Study the drawing (mm; zero at the part's minimum x, y, z) and answer. A direction names the side the tool comes from. Coordinates: 2 decimals unless noted, no trailing zeros. Order: outer loops, then holes, each group sorted by start corner. A loop starts at its lowest first (then second) coordinate and runs counter-clockwise, first axis right, second up. Notation, with made-up numbers: M 56,13.25 L 74,13.25 A22 ccw 74,20.25 Z; hole C -31.75,65.5 d11. An arc over 180 degrees is marked long. Use a Markdown table: item, result. Add a question column.
1) Find section B-B on x = 7.7. Write down the section's boundary in (y, z).
2) Each of these flat-tipped pins is pushed along its axis until it touches: pin 1 Ø3 at (x, y) = (6, 2.5) entering from -Z; pin 2 Ø2.5 at (y, z) = (7, 7) entering from -X; pin 3 Ø2 at (y, z) = (4.5, 7) entering from +X; pin 4 Ø0.5 at (x, z) = (7.5, 2) entering from +Y. Where does it stop, or does it pass through?
3) The mould has two halves that part along Z. Classify the marked faces 4, 5 and 6: released by +Z, released by -Z, zero draft, split by the parting line, or undercut.
4) Find section A-A on z = 1.25. Write down the section's boundary in (x, y).
5) Find the intervals of material crossed by probe 1 along Y at (x, z) = (7.7, 1); probe 2 along X at (y, z) = (5, 2.75); probe 3 along Y at (x, z) = (8.25, 0.75), in increasing order. Write a range as [from, to].
6) Find section D-D on z = 9.3. Write down the section's boundary in (x, y).
7) Find section C-C on y = 2.5. Write down the section's boundary in (x, z), plus the area to 3 significant figures.
8) For the marked faces 1, 2 and 3, determine the directions among +Z, -Z, +X, -X, +Y, -Y from which every point of the face is accessible in a straight line to the end or side of a thin tool.
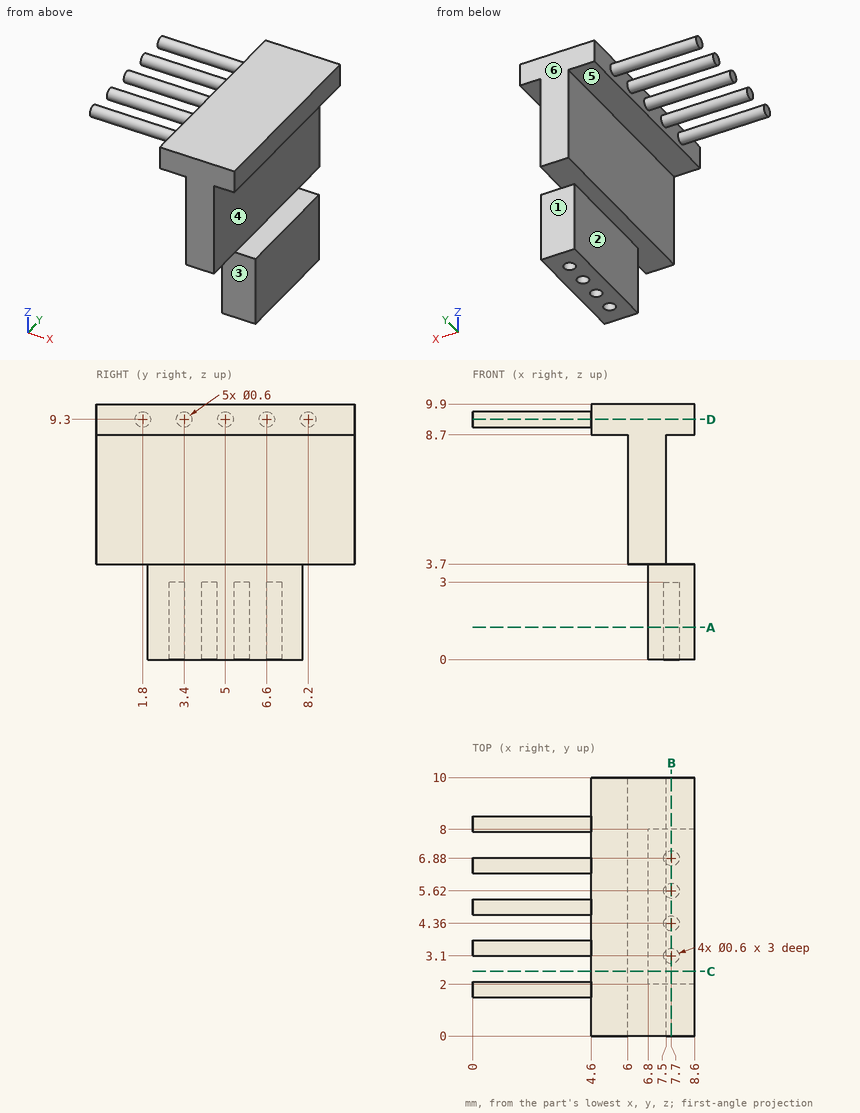
Check result:
| question | item | result |
|---|---|---|
| 1 | outline | M 0,8.7 L 10,8.7 L 10,9.9 L 0,9.9 Z; M 2,0 L 2.8,0 L 2.8,3 L 3.4,3 L 3.4,0 L 4.06,0 L 4.06,3 L 4.66,3 L 4.66,0 L 5.32,0 L 5.32,3 L 5.92,3 L 5.92,0 L 6.58,0 L 6.58,3 L 7.18,3 L 7.18,0 L 8,0 L 8,3.7 L 2,3.7 Z |
| 2 | pin 1 | stops at z = 0 |
| 2 | pin 2 | stops at x = 6 |
| 2 | pin 3 | stops at x = 7.5 |
| 2 | pin 4 | stops at y = 8 |
| 3 | face 4 | undercut |
| 3 | face 5 | released by -Z |
| 3 | face 6 | zero draft |
| 4 | outline | M 6.8,2 L 8.6,2 L 8.6,8 L 6.8,8 Z; hole C 7.7,3.1 d0.6; hole C 7.7,4.36 d0.6; hole C 7.7,5.62 d0.6; hole C 7.7,6.88 d0.6 |
| 5 | probe 1 | y = [2, 2.8], [3.4, 4.06], [4.66, 5.32], [5.92, 6.58], [7.18, 8] |
| 5 | probe 2 | x = [6.8, 8.6] |
| 5 | probe 3 | y = [2, 8] |
| 6 | outline | M 0,1.5 L 4.6,1.5 L 4.6,0 L 8.6,0 L 8.6,10 L 4.6,10 L 4.6,8.5 L 0,8.5 L 0,7.9 L 4.6,7.9 L 4.6,6.9 L 0,6.9 L 0,6.3 L 4.6,6.3 L 4.6,5.3 L 0,5.3 L 0,4.7 L 4.6,4.7 L 4.6,3.7 L 0,3.7 L 0,3.1 L 4.6,3.1 L 4.6,2.1 L 0,2.1 Z |
| 7 | outline | M 4.6,8.7 L 6,8.7 L 6,3.7 L 6.8,3.7 L 6.8,0 L 8.6,0 L 8.6,3.7 L 7.5,3.7 L 7.5,8.7 L 8.6,8.7 L 8.6,9.9 L 4.6,9.9 Z |
| 7 | area | 19.0 mm2 |
| 8 | face 1 | -Z, +X, -X, +Y |
| 8 | face 2 | -Z, -X, +Y, -Y |
| 8 | face 3 | -Z, +X, -X, -Y |
